```python
from build123d import *

# Parameters (mm, degrees)
EXTRUDE_THIN1_DEPTH               = 4.075
CUT_EXTRUDE1_DEPTH                = 8.45230669
CUT_EXTRUDE1_DEPTH_BACK           = 8.45230669
BOSS_EXTRUDE1_DEPTH               = 1
BOSS_EXTRUDE2_DEPTH               = 0.5
BOSS_EXTRUDE2_DEPTH_BACK          = 5
SKETCH5_R                         = 2
SKETCH6_R                         = 3.35
BOSS_EXTRUDE3_DEPTH               = 2
FILLET1_R                         = 0.75
SKETCH7_W                         = 1.15
SKETCH7_H                         = 5.2
CUT_EXTRUDE_THIN1_DEPTH           = 2
CUT_EXTRUDE_THIN1_DRAFT           = -13
SKETCH7_W_2                       = 3.5
SKETCH7_H_2                       = 1.15
CUT_EXTRUDE_THIN1_PROFILE_2_DEPTH = 2
CUT_EXTRUDE_THIN1_PROFILE_2_DRAFT = -13


with BuildPart() as part:
    # Sketch1 → Extrude-Thin1 (new, symmetric)
    with BuildSketch(Plane(origin=(0, 0, 0), x_dir=(0, 0, -1), z_dir=(1, 0, 0))):
        with BuildLine():
            Line((-4.075, -3.725), (-4.075, 3.725))
            ThreePointArc((-4.075, 3.725), (-3.782106781, 4.432106781), (-3.075, 4.725))
            Line((-3.075, 4.725), (3.075, 4.725))
            ThreePointArc((3.075, 4.725), (3.782106781, 4.432106781), (4.075, 3.725))
            Line((4.075, 3.725), (4.075, -3.725))
            Line((4.075, -3.725), (3.225, -3.725))
            Line((3.225, -3.725), (3.225, 3.725))
            ThreePointArc((3.225, 3.725), (3.181066017, 3.831066017), (3.075, 3.875))
            Line((3.075, 3.875), (-3.075, 3.875))
            ThreePointArc((-3.075, 3.875), (-3.181066017, 3.831066017), (-3.225, 3.725))
            Line((-3.225, 3.725), (-3.225, -3.725))
            Line((-3.225, -3.725), (-4.075, -3.725))
        make_face()
    extrude(amount=EXTRUDE_THIN1_DEPTH, both=True)

    # Sketch3 → Cut-Extrude1 (cut, two sides: drawn at the far end of the back side and taken through both)
    with BuildSketch(Plane.XY.offset(-CUT_EXTRUDE1_DEPTH_BACK)):
        with BuildLine():
            Line((-1.715, -3.725), (1.715, -3.725))
            Line((1.715, -3.725), (1.715, -3.972782835))
            Line((1.715, -3.972782835), (3.215, -3.972782835))
            Line((3.215, -3.972782835), (3.215, -3.725))
            Line((3.215, -3.725), (4.075, -3.725))
            Line((4.075, -3.725), (4.075, 0.775))
            ThreePointArc((4.075, 0.775), (3.466888168, 0.523111832), (3.215, -0.085))
            Line((3.215, -0.085), (3.215, -2.975))
            ThreePointArc((3.215, -2.975), (2.465, -3.725), (1.715, -2.975))
            Line((1.715, -2.975), (1.715, 1.775))
            ThreePointArc((1.715, 1.775), (1.568553391, 2.128553391), (1.215, 2.275))
            Line((1.215, 2.275), (-1.215, 2.275))
            ThreePointArc((-1.215, 2.275), (-1.568553391, 2.128553391), (-1.715, 1.775))
            Line((-1.715, 1.775), (-1.715, -2.975))
            ThreePointArc((-1.715, -2.975), (-2.465, -3.725), (-3.215, -2.975))
            Line((-3.215, -2.975), (-3.215, -0.085))
            ThreePointArc((-3.215, -0.085), (-3.466888168, 0.523111832), (-4.075, 0.775))
            Line((-4.075, 0.775), (-4.075, -3.725))
            Line((-4.075, -3.725), (-3.215, -3.725))
            Line((-3.215, -3.725), (-3.215, -3.972782835))
            Line((-3.215, -3.972782835), (-1.715, -3.972782835))
            Line((-1.715, -3.972782835), (-1.715, -3.725))
        make_face()
    extrude(amount=CUT_EXTRUDE1_DEPTH + CUT_EXTRUDE1_DEPTH_BACK, mode=Mode.SUBTRACT)

    # Sketch4 → Boss-Extrude1 (add)
    with BuildSketch(Plane(origin=(0, 4.725, 0), x_dir=(1, 0, 0), z_dir=(0, 1, 0))):
        with BuildLine():
            Line((-2.7, -3.7), (2.7, -3.7))
            ThreePointArc((2.7, -3.7), (3.407106781, -3.407106781), (3.7, -2.7))
            Line((3.7, -2.7), (3.7, 2.7))
            ThreePointArc((3.7, 2.7), (3.407106781, 3.407106781), (2.7, 3.7))
            Line((2.7, 3.7), (-2.7, 3.7))
            ThreePointArc((-2.7, 3.7), (-3.407106781, 3.407106781), (-3.7, 2.7))
            Line((-3.7, 2.7), (-3.7, -2.7))
            ThreePointArc((-3.7, -2.7), (-3.407106781, -3.407106781), (-2.7, -3.7))
        make_face()
    extrude(amount=BOSS_EXTRUDE1_DEPTH)

    # Sketch5 → Boss-Extrude2 (add, two sides: drawn at the far end of the back side and taken through both)
    with BuildSketch(Plane(origin=(0, 5.725, 0), x_dir=(1, 0, 0), z_dir=(0, 1, 0)).offset(-BOSS_EXTRUDE2_DEPTH_BACK)):
        with Locations(Location((0, 0, 0), (0, 0, 270))):
            Circle(SKETCH5_R)
    extrude(amount=BOSS_EXTRUDE2_DEPTH + BOSS_EXTRUDE2_DEPTH_BACK)

    # Sketch6 → Boss-Extrude3 (add)
    with BuildSketch(Plane(origin=(0, 6.225, 0), x_dir=(1, 0, 0), z_dir=(0, 1, 0))):
        with Locations(Location((0, 0, 0), (0, 0, 270))):
            Circle(SKETCH6_R)
    extrude(amount=BOSS_EXTRUDE3_DEPTH)

    # Fillet1
    fillet1_edges = [part.edges().sort_by_distance(p)[0] for p in [
        (0, 6.225, -3.35),
        (0, 8.225, -3.35),
    ]]
    fillet(fillet1_edges, radius=FILLET1_R)


with BuildPart() as cut_extrude_thin1_tool:
    # Sketch7 → Cut-Extrude-Thin1 (with draft: the straight prism first)
    with BuildSketch(Plane(origin=(0, 8.225, 0), x_dir=(1, 0, 0), z_dir=(0, 1, 0))):
        Rectangle(SKETCH7_W, SKETCH7_H)
    extrude(amount=-CUT_EXTRUDE_THIN1_DEPTH)
    # Cut-Extrude-Thin1: the draft: its side faces are tilted about the plane it starts from
    cut_extrude_thin1_sides = [cut_extrude_thin1_tool.faces().sort_by_distance(p)[0] for p in [
        (-0.575, 7.225, 0),
        (0, 7.225, 2.6),
        (0.575, 7.225, 0),
        (0, 7.225, -2.6),
    ]]
    draft(cut_extrude_thin1_sides, Plane(origin=(0, 8.225, 0), x_dir=(1, 0, 0), z_dir=(0, 1, 0)), CUT_EXTRUDE_THIN1_DRAFT)


with BuildPart() as part_1:
    add(part.part)

    # Cut-Extrude-Thin1: cut by cut_extrude_thin1_tool
    add(cut_extrude_thin1_tool.part, mode=Mode.SUBTRACT)


with BuildPart() as cut_extrude_thin1_profile_2_tool:
    # Sketch7 → Cut-Extrude-Thin1 profile 2 (with draft: the straight prism first)
    with BuildSketch(Plane(origin=(0, 8.225, 0), x_dir=(1, 0, 0), z_dir=(0, 1, 0))):
        Rectangle(SKETCH7_W_2, SKETCH7_H_2)
    extrude(amount=-CUT_EXTRUDE_THIN1_PROFILE_2_DEPTH)
    # Cut-Extrude-Thin1 profile 2: the draft: its side faces are tilted about the plane it starts from
    cut_extrude_thin1_profile_2_sides = [cut_extrude_thin1_profile_2_tool.faces().sort_by_distance(p)[0] for p in [
        (0, 7.225, -0.575),
        (-1.75, 7.225, 0),
        (0, 7.225, 0.575),
        (1.75, 7.225, 0),
    ]]
    draft(cut_extrude_thin1_profile_2_sides, Plane(origin=(0, 8.225, 0), x_dir=(1, 0, 0), z_dir=(0, 1, 0)), CUT_EXTRUDE_THIN1_PROFILE_2_DRAFT)


with BuildPart() as part_2:
    add(part_1.part)

    # Cut-Extrude-Thin1 profile 2: cut by cut_extrude_thin1_profile_2_tool
    add(cut_extrude_thin1_profile_2_tool.part, mode=Mode.SUBTRACT)


solid = part_2.part
```
Check sheet for the modelled part. Datum: model origin and axes. Units: mm. A direction names the side the tool comes from. Coordinates: 2 decimals unless noted, no trailing zeros. Order: outer loops, then holes, each group sorted by start corner. A loop starts at its lowest first (then second) coordinate and runs counter-clockwise, first axis right, second up. Notation, with made-up numbers: M 10.5,31.25 L 66.5,31.25 A33 cw 66.5,64.25 Z; hole C 63,1.25 d9. An arc over 180 degrees is marked long. Write each question's results on one line, items separated by ' | '. Start each with the question number.
1. Cross-section at D-D on y = 2. Record the cut outline in (x, z) (3 decimals).
2. Go/stop test with flat-tipped pins: P1, Ø4, axis at y = 7, z = 3, coming from the -X side; P2, Ø1.6, axis at x = 0, z = -1, coming from the -Y side (3 decimals); P3, Ø2, axis at x = 3, z = -2.5, coming from the +Y side. Record where each tip stops, or that it passes through.
3. Material ranges on probe 1 along Y at (x, z) = (2, 1.75) (3 decimals); probe 2 along Z at (x, y) = (-2.5, 1) (3 decimals); probe 3 along Y at (x, z) = (1, 1.5) (3 decimals), recorded low to high.
4. Cross-section at C-C on y = 7.25. Record the cut outline in (x, z).
5. Cross-section at B-B on z = 3.5. Record the cut outline in (x, y) (3 decimals), and give its area (3 significant figures).
6. Access from +Z, -Z, +X, -X, +Y, -Y to the whole of each face (thin tool, end or side, straight path). Record for faces 1 (the face through (0, 5, -3.7)), 2 (the face through (1.715, -0.6, -3.7)), 3 (the face through (0.92, 7.239, 0.347)).
7. Cross-section at A-A on y = -2.25. Record the cut outline in (x, z) (3 decimals).
Checks:
1) outline: M -4.075,-4.075 L -1.662,-4.075 L -1.662,-3.225 L -4.075,-3.225 Z; M -4.075,3.225 L -1.662,3.225 L -1.662,4.075 L -4.075,4.075 Z; C 0,0 d4; M 1.662,-4.075 L 4.075,-4.075 L 4.075,-3.225 L 1.662,-3.225 Z; M 1.662,3.225 L 4.075,3.225 L 4.075,4.075 L 1.662,4.075 Z
2) P1: stops at x = -3.7 | P2: stops at y = 0.725 | P3: stops at y = 8.16
3) probe 1: y = 3.875 to 5.725, 6.227 to 8.223 | probe 2: z = -4.075 to -3.225, 3.225 to 4.075 | probe 3: y = 0.725 to 8.225
4) outline: C 0,0 d6.7; hole M -1.52,-0.35 L -0.35,-0.35 L -0.35,-2.37 L 0.35,-2.37 L 0.35,-0.35 L 1.52,-0.35 L 1.52,0.35 L 0.35,0.35 L 0.35,2.37 L -0.35,2.37 L -0.35,0.35 L -1.52,0.35 Z
5) outline: M -4.075,0.775 A0.86 cw -3.215,-0.085 L -3.215,-2.975 A0.75 ccw -1.715,-2.975 L -1.715,1.775 A0.5 cw -1.215,2.275 L 1.215,2.275 A0.5 cw 1.715,1.775 L 1.715,-2.975 A0.75 ccw 3.215,-2.975 L 3.215,-0.085 A0.86 cw 4.075,0.775 L 4.075,4.63 L -4.075,4.63 Z; M -3.3,4.725 L 3.3,4.725 L 3.3,5.725 L -3.3,5.725 Z | area: 46.3 mm²
6) face 1: -Z, +X, -X, +Y | face 2: -Z, -Y | face 3: +Y
7) outline: M -3.215,-4.075 L -1.715,-4.075 L -1.715,-3.225 L -3.215,-3.225 Z; M -3.215,3.225 L -1.715,3.225 L -1.715,4.075 L -3.215,4.075 Z; M 1.715,-4.075 L 3.215,-4.075 L 3.215,-3.225 L 1.715,-3.225 Z; M 1.715,3.225 L 3.215,3.225 L 3.215,4.075 L 1.715,4.075 Z
